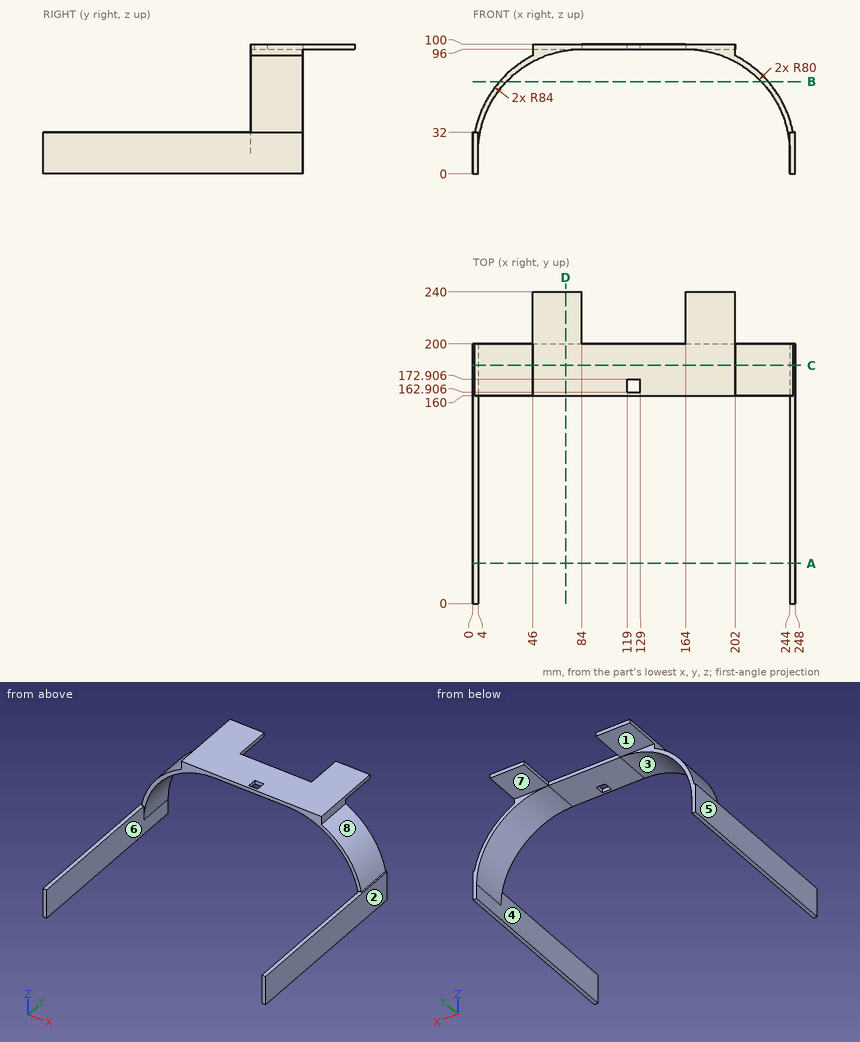
For this review, use the dimensioned drawing (mm, ordinates from the lowest corner) and the shaded views. A direction names the side the tool comes from. Give positions to 0.01 mm unless a question says otherwise; leave off trailing zeros. Order: outer loops, then holes, each group sorted by start corner. A loop starts at its lowest first (then second) coordinate and runs counter-clockwise, first axis right, second up. Notation, with made-up numbers: M -31,-22 L -12,-22 A18 ccw -12,-10 Z; hole C -40,-27.5 d8. An arc over 180 degrees is marked long. One line per question, with ' | ' between items. Start each with the question number.
1) Clearance check with flat-ended pins moving along their axes: P1, Ø2, axis at x = 133, z = 97, coming from the +Y side; P2, Ø3, axis at x = 1.5, y = 145, coming from the +Z side; P3, Ø12, axis at x = 37.5, y = 208.5, coming from the -Z side; P4, Ø12, axis at x = 134, y = 190, coming from the -Z side. State where each tip first meets the part, or that it passes through.
2) Wall thickness on L1, parallel to Z at x = 183.5, y = 201.5; L2, parallel to X at y = 155.5, z = 10; L3, parallel to X at y = 180, z = 39: over which ranges is each line inside the solid? List them lowest first. Write a range as from..to.
3) Mouldability with a two-part tool opening along X and no side actions: class the marked faces 6, 7 and 8 as pulls with the +X half, pulls with the -X half, needs draft (parallel to the pull), parting line crosses it, or undercut.
4) Consider section D-D, the plane x = 71.5. Give the boundary of the cut face in (y, z).
5) Consider section B-B, the plane z = 71. Give the boundary of the cut face in (x, y), then the cut area to 3 significant figures.
6) Consider section A-A, the plane y = 31. Give the boundary of the cut face in (x, z).
7) For the marked faces 1, 2, 3, 4 and 5, list the 3-axis set-ups (+Z, -Z, +X, -X, +Y, -Y) from which the entire face can be reached by the end or side of a thin tool; tool diameter is ignored.
8) Consider section C-C, the plane y = 183.5. Give the boundary of the cut face in (x, z), then the cut area to 3 significant figures.
Found:
1) P1: stops at y = 200 | P2: stops at z = 32 | P3: passes through | P4: stops at z = 96
2) L1: z = 96..100 | L2: x = 0..4, 244..248 | L3: x = 3.21..7.38, 240.62..244.79
3) face 6: undercut | face 7: needs draft | face 8: pulls with the +X half
4) outline: M 160,95.02 L 200,95.02 L 200,96 L 240,96 L 240,100 L 160,100 Z
5) outline: M 20.51,160 L 25.91,160 L 25.91,200 L 20.51,200 Z; M 222.09,160 L 227.49,160 L 227.49,200 L 222.09,200 Z | area: 432 mm²
6) outline: M 0,0 L 4,0 L 4,32 L 0,32 Z; M 244,0 L 248,0 L 248,32 L 244,32 Z
7) face 1: -Z, +X, -X, +Y | face 2: +Z, -Z, +X, +Y, -Y | face 3: -Z, +Y, -Y | face 4: -Z, -Y | face 5: +Z, -Z, -X, +Y, -Y
8) outline: M 0,0 L 4,0 L 4,16 A80 cw 84,96 L 164,96 A80 cw 244,16 L 244,0 L 248,0 L 248,32 L 246.46,32 A84 ccw 202,90.91 L 202,100 L 46,100 L 46,90.91 A84 ccw 1.54,32 L 0,32 Z | area: 1,720 mm²
